Autodesk Inventor part; units mm, degrees
ref_plane "YZ Plane" through (0, 0, 0) normal (1, 0, 0) x (0, 1, 0)
ref_plane "XZ Plane" through (0, 0, 0) normal (0, 1, 0) x (-1, 0, 0)
ref_plane "XY Plane" through (0, 0, 0) normal (0, 0, 1) x (1, 0, 0)
sketch "Sketch1" plane through (0, 0, 0) normal (0, 0, 1) x (1, 0, 0)
  arc A0 (15.5, 0) -> (-15.5, 0) centre (0, 0) ccw
  line L0 (-15.5, 0) -> (-15.5, -34)
  line L1 (-15.5, -34) -> (15.5, -34)
  line L2 (15.5, -34) -> (15.5, 0)
  circle A1 centre (0, 5) radius 1.85
  circle A2 centre (-5, 0) radius 1.85
  circle A3 centre (0, -5) radius 1.85
  circle A4 centre (5, 0) radius 1.85
  dimension "d0" = 31
  dimension "d1" = 34
  dimension "d3" = 3.7
  dimension "d6" = 360
extrude "Extrusion1" add sketch "Sketch1" along normal blind 5
sketch "Sketch2" plane through (0, 0, 5) normal (0, 0, 1) x (1, 0, 0)
  line L0 (-15.5, -34) -> (15.5, -34)
  line L1 (15.5, -34) -> (15.5, 0)
  line L2 (-15.5, -34) -> (15.5, -34)
  line L3 (15.5, -34) -> (15.5, -31)
  line L4 (15.5, -31) -> (-15.5, -31)
  line L5 (-15.5, -31) -> (-15.5, -34)
  point P0 (0, 0)
  dimension "d10" = 3
extrude "Extrusion2" add sketch "Sketch2" along normal blind 22
sketch "Sketch3" plane through (0, 0, 27) normal (0, 0, 1) x (1, 0, 0)
  line L0 (15.5, -31) -> (-15.5, -31)
  line L1 (15.5, -34) -> (15.5, 0)
  line L2 (15.5, -31) -> (15.5, 0)
  line L3 (-15.5, 0) -> (-15.5, -31)
  line L4 (-15.5, 0) -> (-15.5, -31)
  line L5 (-15.5, -31) -> (15.5, -31)
  arc A0 (15.5, 0) -> (-15.5, 0) centre (0, 0) ccw
  point P0 (0, 0)
extrude "Extrusion3" add sketch "Sketch3" against normal blind 4
sketch "Sketch4" plane through (0, 0, 0) normal (0, 0, -1) x (-1, 0, 0)
  circle A0 centre (0, 0) radius 3.75
  dimension "d15" = 7.5
extrude "Extrusion4" add sketch "Sketch4" along normal blind 6
sketch "Sketch5" plane through (0, 0, 27) normal (0, 0, 1) x (1, 0, 0)
  circle A0 centre (0, 0) radius 3.75
  dimension "d20" = 7.5
extrude "Extrusion5" add sketch "Sketch5" along normal blind 6
sketch "Sketch6" plane through (-15.5, -31, 5) normal (0, 1, 0) x (1, 0, 0)
  line L0 (0, -18) -> (31, -18)
  line L1 (17.35, 0) -> (13.65, 0)
  circle A0 centre (9.5, -9) radius 1.625
  circle A1 centre (15.5, -15) radius 1.625
  circle A2 centre (21.5, -9) radius 1.625
  circle A3 centre (15.5, -3) radius 1.625
  point P0 (15.5, 5)
  point P1 (15.5, -9)
  dimension "d22" = 3.25
  dimension "d25" = 360
extrude "Extrusion6" cut sketch "Sketch6" against normal through all
sketch "Sketch7" plane through (0, 0, 27) normal (0, 0, 1) x (1, 0, 0)
  circle A0 centre (0, 5) radius 1.625
  circle A1 centre (5, 0) radius 1.625
  circle A2 centre (0, -5) radius 1.625
  circle A3 centre (-5, 0) radius 1.625
  point P0 (0, 0)
  dimension "d31" = 3.25
  dimension "d32" = 3.25
  dimension "d33" = 3.25
  dimension "d34" = 3.25
extrude "Extrusion7" cut sketch "Sketch7" against normal up to surface (4 mm away)
properties part number "Base_Mount"
Part model, mm, in its own coordinate system. A direction names the side the tool comes from. Coordinates: 2 decimals unless noted, no trailing zeros. Loops run counter-clockwise (first coordinate to the right, second up) from the corner with the lowest first, then second, coordinate; pieces in that order, holes last. Notation, with made-up numbers: (-2.5, -16.5) -> (45.5, -16.5) arc R17 cw to (45.5, 8.5) -> close; hole circle Ø6 at (15, 88). An arc over 180 degrees is marked (long way). Use a Markdown table: item, result. Add a question column.
Item 1: Band-saw the part on A-A on y = -18. Write the cut outline in (x, z), plus the area to 3 significant figures.
Item 2: Probe probe 1 along X at (y, z) = (-32, 14) (3 decimals); probe 2 along Y at (x, z) = (0, 25.55) (3 decimals); probe 3 along Z at (x, y) = (9.5, -24.5). List the from-to ranges inside material, lowest first.
Item 3: Band-saw the part on B-B on z = 24.5. Write the cut outline in (x, y) (3 decimals).
Item 4: Band-saw the part on D-D on x = 5. Write the cut outline in (y, z) (3 decimals).
Item 5: Pull direction Y, two halves, no side cores. Call faces 6 (the cylindrical face through (0.341, 15.496, 25.028)), 7 (the cylindrical face through (-6.623, 0.071, 25.028)), 8 (the flat face through (0, -34, 13)): +Y half, -Y half, draft (parallel to the pull), parting line (faces both ways), or undercut.
Item 6: Band-saw the part on C-C on z = 8. Write the cut outline in (x, y) (3 decimals), plus the area to 4 significant figures.
Item 7: Which spindle directions (+Z, -Z, +X, -X, +Y, -Y) get a long thin tool onto all of the face, cutting with end or side? Do faces 1 (the flat face through (0, -7, 23)), 2 (the cylindrical face through (3.746, -0.165, -2.958)), 3 (the cylindrical face through (-3.746, -0.165, 29.958)), 4 (the cylindrical face through (-0.341, 15.496, 2.465)), 5 (the cylindrical face through (-0.241, 3.166, 2.465)). Say none if no direction does.
Item 8: Flat gauge pins, fed straight in: P1, Ø5, axis at y = 8.5, z = 27.5, coming from the -X side; P2, Ø12, axis at y = 7, z = 20, coming from the +X side; P3, Ø12, axis at x = 5, y = -20.5, coming from the +Z side; P4, Ø1.9, axis at x = 0, y = 5, coming from the +Z side. Where does each tip first touch, or does it go through?
Geometry says:
| question | item | result |
|---|---|---|
| 1 | outline | (-15.5, 0) -> (15.5, 0) -> (15.5, 5) -> (-15.5, 5) -> close; (-15.5, 23) -> (15.5, 23) -> (15.5, 27) -> (-15.5, 27) -> close |
| 1 | area | 279 mm² |
| 2 | probe 1 | -15.5 to -7.625, -4.375 to 4.375, 7.625 to 15.5 |
| 2 | probe 2 | -34 to -6.625, -3.375 to 3.375, 6.625 to 15.5 |
| 2 | probe 3 | 0 to 5, 23 to 27 |
| 3 | outline | (-15.5, -34) -> (15.5, -34) -> (15.5, 0) arc R15.5 ccw to (-15.5, 0) -> close; hole circle Ø3.25 at (-5, 0); hole circle Ø3.25 at (0, -5); hole circle Ø3.25 at (0, 5); hole circle Ø3.25 at (5, 0) |
| 4 | outline | (-34, 0) -> (-1.85, 0) -> (-1.85, 5) -> (-31, 5) -> (-31, 12.719) -> (-34, 12.719) -> close; (-34, 15.281) -> (-31, 15.281) -> (-31, 23) -> (-1.625, 23) -> (-1.625, 27) -> (-34, 27) -> close; (1.625, 23) -> (14.671, 23) -> (14.671, 27) -> (1.625, 27) -> close; (1.85, 0) -> (14.671, 0) -> (14.671, 5) -> (1.85, 5) -> close |
| 5 | face 6 | +Y half |
| 5 | face 7 | undercut |
| 5 | face 8 | -Y half |
| 6 | outline | (-15.5, -34) -> (-1.625, -34) -> (-1.625, -31) -> (-15.5, -31) -> close; (1.625, -34) -> (15.5, -34) -> (15.5, -31) -> (1.625, -31) -> close |
| 6 | area | 83.25 mm² |
| 7 | face 1 | +X, -X, +Y |
| 7 | face 2 | -Z |
| 7 | face 3 | +Z |
| 7 | face 4 | +Z, -Z, +Y |
| 7 | face 5 | none |
| 8 | P1 | x = -14.27 |
| 8 | P2 | x = 15.39 |
| 8 | P3 | z = 27 |
| 8 | P4 | through |
